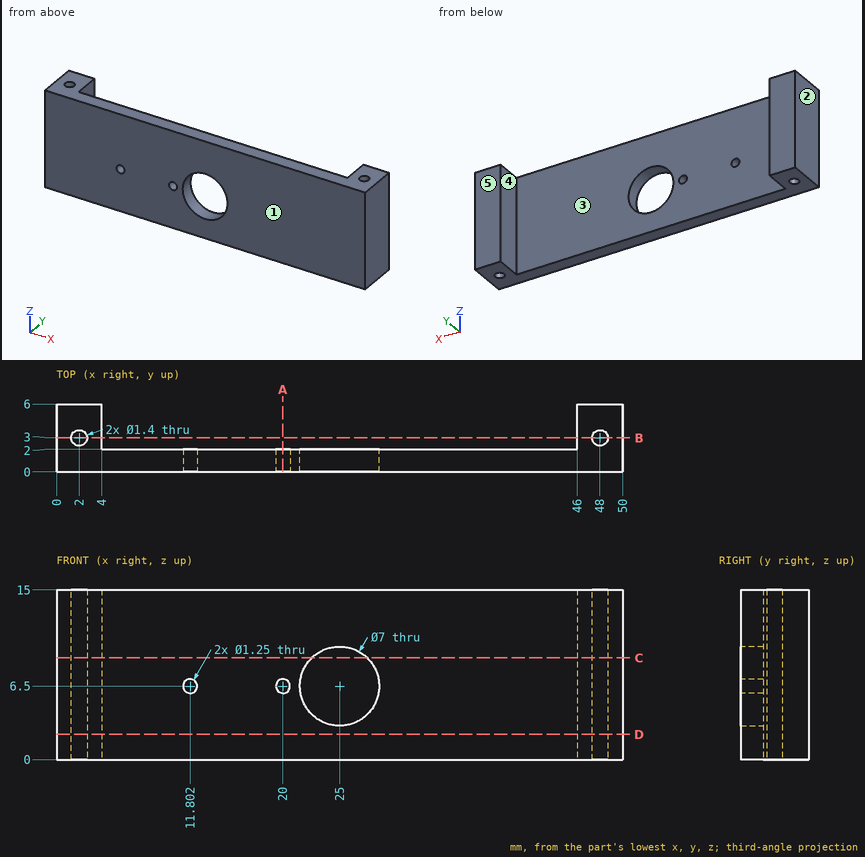
Part print with two shaded views. Sizes in mm from the minimum x, y, z corner. A direction names the side the tool comes from. Give positions to 0.01 mm unless a question says otherwise; leave off trailing zeros. Order: outer loops, then holes, each group sorted by start corner. A loop starts at its lowest first (then second) coordinate and runs counter-clockwise, first axis right, second up.
1) Saw through at D-D, the plane z = 2.25. Write the cut outline in (x, y).
2) Pin check, flat tip, straight feed: pin 1 (2 mm diameter, centred on x = 25, z = 12.5, fed in from +Y). Stop position of the tip, or through.
3) Saw through at C-C, the plane z = 9. Write the cut outline in (x, y), then the cut area to 3 significant figures.
4) 3-axis set-ups, long thin cutter, end or side, ignore diameter. For the marked faces 4 and 5: which of +Z, -Z, +X, -X, +Y, -Y reach the whole face in a straight line?
5) Mould opens along X. For the marked faces 1, 2 and 3 say: +X half, -X half, draft (parallel to the pull), parting line (faces both ways), or undercut.
6) Saw through at A-A, the plane x = 20. Write the cut outline in (y, z) (1 decimal).
7) Saw through at B-B, the plane y = 3. Write the cut outline in (x, z).
8) Wall check: probe 1 along X at (y, z) = (1.45, 6.5) (1 decimal); probe 2 along X at (y, z) = (2.85, 3.75); probe 3 along X at (y, z) = (4.8, 6.25). Give the ranges that are in metal, low to high.
Computed:
1. outline: (0, 0) - (50, 0) - (50, 6) - (46, 6) - (46, 2) - (4, 2) - (4, 6) - (0, 6) - close; hole circle Ø1.4 at (2, 3); hole circle Ø1.4 at (48, 3)
2. pin 1: stops at y = 2
3. outline: (0, 0) - (22.55, 0) - (22.55, 2) - (4, 2) - (4, 6) - (0, 6) - close; (27.45, 0) - (50, 0) - (50, 6) - (46, 6) - (46, 2) - (27.45, 2) - close; hole circle Ø1.4 at (2, 3); hole circle Ø1.4 at (48, 3)
3. area: 119 mm2
4. face 4: +Z, -Z, +Y
4. face 5: +Z, -Z, +X, -X, +Y
5. face 1: draft
5. face 2: -X half
5. face 3: undercut
6. outline: (0, 0) - (2, 0) - (2, 5.9) - (0, 5.9) - close; (0, 7.1) - (2, 7.1) - (2, 15) - (0, 15) - close
7. outline: (0, 0) - (1.3, 0) - (1.3, 15) - (0, 15) - close; (2.7, 0) - (4, 0) - (4, 15) - (2.7, 15) - close; (46, 0) - (47.3, 0) - (47.3, 15) - (46, 15) - close; (48.7, 0) - (50, 0) - (50, 15) - (48.7, 15) - close
8. probe 1: x = 0 to 11.2, 12.4 to 19.4, 20.6 to 21.5, 28.5 to 50
8. probe 2: x = 0 to 1.32, 2.68 to 4, 46 to 47.32, 48.68 to 50
8. probe 3: x = 0 to 4, 46 to 50
